from build123d import *

# Parameters (mm, degrees)
SKETCH1_R                 = 28.575
SKETCH1_R_2               = 20.955
BOSS_EXTRUDE1_DEPTH       = 1.96215
BOSS_EXTRUDE1_DEPTH_BACK  = 1.96215
F_0_80_TAPPED_HOLE1_D     = 1.19126
F_0_80_TAPPED_HOLE1_DEPTH = 3.302
F_0_80_TAPPED_HOLE1_TIP   = 0.357890611
SKETCH4_R                 = 25.4
SKETCH4_R_2               = 22.225
CUT_EXTRUDE2_DEPTH        = 3.175
CUT_EXTRUDE3_DEPTH        = 3.175
CIRPATTERN1_COUNT         = 8


with BuildPart() as part:
    # Sketch1 → Boss-Extrude1 (new body, two sides)
    with BuildSketch(Plane.XY) as boss_extrude1_sk:
        Circle(SKETCH1_R)
        Circle(SKETCH1_R_2, mode=Mode.SUBTRACT)
    extrude(amount=BOSS_EXTRUDE1_DEPTH)
    extrude(boss_extrude1_sk.sketch, amount=-BOSS_EXTRUDE1_DEPTH_BACK)

    # #0-80 Tapped Hole1
    with Locations(Plane(origin=(0, 28.575, 0.041948097), x_dir=(1, 0, 0), z_dir=(0, 1, 0))):
        with Locations((0, 0)):
            Hole(F_0_80_TAPPED_HOLE1_D / 2, depth=F_0_80_TAPPED_HOLE1_DEPTH)
            with Locations((0, 0, -(F_0_80_TAPPED_HOLE1_DEPTH + F_0_80_TAPPED_HOLE1_TIP / 2))):  # 118° drill point
                Cone(0, F_0_80_TAPPED_HOLE1_D / 2, F_0_80_TAPPED_HOLE1_TIP, mode=Mode.SUBTRACT)

    # Sketch4 → Cut-Extrude2 (cut)
    with BuildSketch(Plane(origin=(0, 0, -1.96215), x_dir=(-1, 0, 0), z_dir=(0, 0, -1))):
        Circle(SKETCH4_R)
        Circle(SKETCH4_R_2, mode=Mode.SUBTRACT)
    extrude(amount=-CUT_EXTRUDE2_DEPTH, mode=Mode.SUBTRACT)

    # Sketch5 → Cut-Extrude3 (cut)
    with BuildSketch(Plane(origin=(0, 0, -1.96215), x_dir=(-1, 0, 0), z_dir=(0, 0, -1))):
        with BuildLine():
            Line((2.54, 31.115), (2.54, 24.765))
            ThreePointArc((2.54, 24.765), (0, 22.225), (-2.54, 24.765))
            Line((-2.54, 24.765), (-2.54, 31.115))
            ThreePointArc((-2.54, 31.115), (0, 33.655), (2.54, 31.115))
        make_face()
    cut_extrude3 = extrude(amount=-CUT_EXTRUDE3_DEPTH, mode=Mode.SUBTRACT)

    # CirPattern1: Cut-Extrude3 ×8 about axis
    cirpattern1_axis = Axis((0, 0, 0), (0, 0, 1))
    for i in range(1, CIRPATTERN1_COUNT):
        add(cut_extrude3.rotate(cirpattern1_axis, i * 360 / CIRPATTERN1_COUNT), mode=Mode.SUBTRACT)


solid = part.part
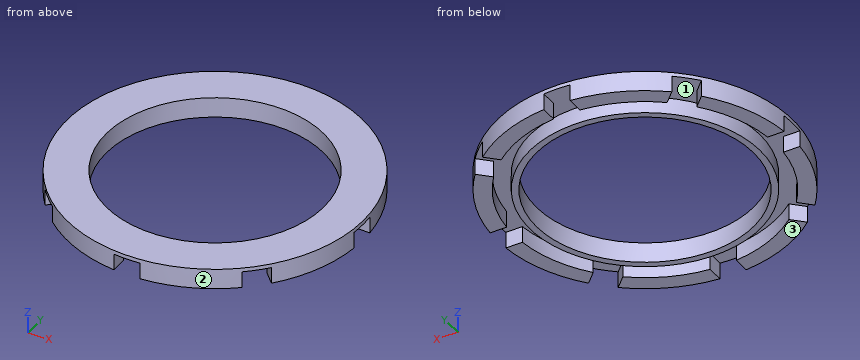
CAD build for the part. Positions are in the model's coordinates, mm. Face numbers are marked on the shaded views. Coordinates: 2 decimals unless noted, no trailing zeros. Loops run counter-clockwise (first coordinate to the right, second up) from the corner with the lowest first, then second, coordinate; pieces in that order, holes last. Notation, with made-up numbers: (-9, 59.25) -> (5, 59.25) arc R37 ccw to (5, 98.25) -> close; hole circle Ø7 at (-21.75, 51). An arc over 180 degrees is marked (long way). One line per item, written item: value.
1. Slice it at A-A on z = 0.45. Give the number of separate pieces and of enclosed holes in the cut face, and give its area (3 significant figures).
Answers:
separate pieces: 9
enclosed holes: 1
area: 581 mm^2
2. Drill centre lines: line 1 (Y direction, x = 0, z = 0.4) (3 decimals); line 2 (Y direction, x = 8.5, z = -0.05); line 3 (X direction, y = 16.5, z = 0). Where is each one in solid material? Low to high. Write a range as [from, to].
Answers:
line 1: y = [-22.225, -20.955], [20.955, 22.225]
line 2: y = [-27.28, -23.94], [-20.54, -19.15], [19.15, 20.54], [23.94, 27.28]
line 3: x = [-23.33, -20.09], [-14.89, -12.92], [12.92, 14.89], [20.09, 23.33]
3. Pull direction Y, two halves, no side cores. Call the marked faces 1, 2 and 3: pulls with the +Y half, pulls with the -Y half, needs draft (parallel to the pull), parting line crosses it, or undercut.
Answers:
face 1: undercut
face 2: parting line crosses it
face 3: needs draft
4. Flat gauge pins, fed straight in: P1, Ø1.6, axis at x = 27, z = 0, coming from the -Y side; P2, Ø1.5, axis at x = 23, z = -1.5, coming from the -Y side; P3, Ø1.6, axis at y = -26.5, z = 0, coming from the -X side. Where does each tip first touch, or does it go through?
Answers:
P1: stops at y = -11.41
P2: stops at y = -17.93
P3: stops at x = -12.49
5. Slice it at D-D on y = 13.5. Write the cut outline in (x, z), and give its area (3 significant figures).
Answers:
outline: (-25.18, -1.96) -> (-21.52, -1.96) -> (-21.52, 1.21) -> (-17.66, 1.21) -> (-17.66, -1.96) -> (-16.03, -1.96) -> (-16.03, 1.96) -> (-25.18, 1.96) -> close; (16.03, -1.96) -> (17.66, -1.96) -> (17.66, 1.21) -> (21.52, 1.21) -> (21.52, -1.96) -> (25.18, -1.96) -> (25.18, 1.96) -> (16.03, 1.96) -> close
area: 47.4 mm^2
6. Slice it at B-B on x = 0. Write the cut outline in (y, z) (3 decimals).
Answers:
outline: (-28.575, 1.213) -> (-22.225, 1.213) -> (-22.225, -1.962) -> (-20.955, -1.962) -> (-20.955, 1.962) -> (-28.575, 1.962) -> close; (20.955, -1.962) -> (22.225, -1.962) -> (22.225, 1.213) -> (28.575, 1.213) -> (28.575, 1.962) -> (20.955, 1.962) -> close
